```python
from build123d import *

# Parameters (mm, degrees)
BRIDA_BASE1_DEPTH         = 4
TALADRO_ROSCADO_M51_D     = 4.2
TALADRO_ROSCADO_M51_DEPTH = 14
TALADRO_ROSCADO_M51_TIP   = 1.2618073


# Sheet-metal steps are written as plain solids
with BuildPart() as part:
    # Croquis1 → Brida base1 (new body)
    with BuildSketch(Plane.XY):
        with BuildLine():
            Line((-19.990811444, 8), (-3.990811444, 8))
            ThreePointArc((-3.990811444, 8), (4.009188556, 0), (-3.990811444, -8))
            Line((-3.990811444, -8), (-19.990811444, -8))
            ThreePointArc((-19.990811444, -8), (-27.990811444, 0), (-19.990811444, 8))
        make_face()
    extrude(amount=-BRIDA_BASE1_DEPTH)

    # Taladro roscado M51
    with Locations(Plane.XY):
        with Locations((-19.990811444, 0), (-3.990811444, 0)):
            Hole(TALADRO_ROSCADO_M51_D / 2, depth=TALADRO_ROSCADO_M51_DEPTH)
            with Locations((0, 0, -(TALADRO_ROSCADO_M51_DEPTH + TALADRO_ROSCADO_M51_TIP / 2))):  # 118° drill point
                Cone(0, TALADRO_ROSCADO_M51_D / 2, TALADRO_ROSCADO_M51_TIP, mode=Mode.SUBTRACT)


solid = part.part
```
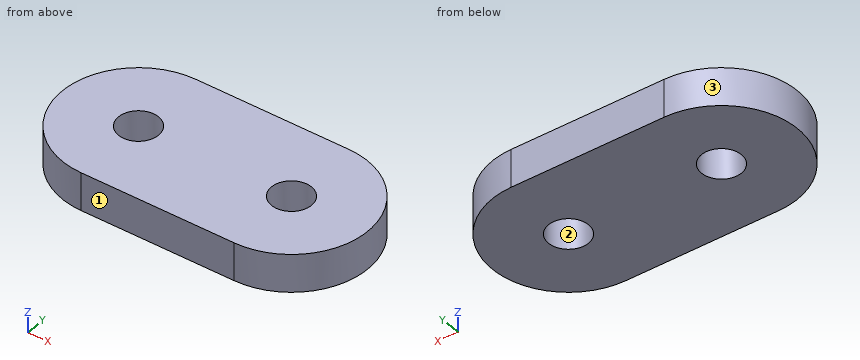
The model under review builds one solid part; all positions refer to its coordinate system, in mm. Face numbers are marked on the shaded views. Give positions to 0.01 mm unless a question says otherwise; leave off trailing zeros. Write each loop counter-clockwise with the first axis right and the second up, starting at its lowest first coordinate (ties: lowest second). Pieces come first, ordered by that corner, then holes. Notation, with made-up numbers: M 72,49.25 L 105,49.25 A25 cw 105,85.25 Z; hole C 55,-0.75 d3. An arc over 180 degrees is marked long. Write each question's results on one line, items separated by ' | '. Start each with the question number.
1. Insertion check: pin 1 Ø5.5 at (x, y) = (-3.99, 0) entering from -Z; pin 2 Ø1 at (y, z) = (5, -3) entering from +X; pin 3 Ø1.5 at (y, z) = (5, -2.5) entering from +X. Each pin has a flat end and moves straight along its axis. Give the tip position at first contact, or say it passes through.
2. We need section D-D (x = -25.5). Write out the cut boundary in (y, z), and give its area (3 significant figures).
3. We need section C-C (x = -5.5). Write out the cut boundary in (y, z).
4. We need section A-A (y = 0). Write out the cut boundary in (x, z), and give its area (3 significant figures).
5. Mouldability with a two-part tool opening along X and no side actions: class the marked faces 1, 2 and 3 as released by +X, released by -X, zero draft, split by the parting line, or undercut.
6. For probe 1 along X at (y, z) = (-0.75, -2.1); probe 2 along Y at (x, z) = (-19.5, -3.6); probe 3 along X at (y, z) = (7, -1.25), list the stretches that pass through material, from the lowest coordinate up. Write a range as [from, to].
7. We need section B-B (z = -2.7). Write out the cut boundary in (x, y), and give its area (3 significant figures).
Results found:
1) pin 1: stops at z = -4 | pin 2: stops at x = 2.62 | pin 3: stops at x = 2.79
2) outline: M -5.8,-4 L 5.8,-4 L 5.8,0 L -5.8,0 Z | area: 46.4 mm^2
3) outline: M -8,-4 L -1.46,-4 L -1.46,0 L -8,0 Z; M 1.46,-4 L 8,-4 L 8,0 L 1.46,0 Z
4) outline: M -27.99,-4 L -22.09,-4 L -22.09,0 L -27.99,0 Z; M -17.89,-4 L -6.09,-4 L -6.09,0 L -17.89,0 Z; M -1.89,-4 L 4.01,-4 L 4.01,0 L -1.89,0 Z | area: 94.4 mm^2
5) face 1: zero draft | face 2: undercut | face 3: released by -X
6) probe 1: x = [-27.96, -21.95], [-18.03, -5.95], [-2.03, 3.97] | probe 2: y = [-8, -2.04], [2.04, 8] | probe 3: x = [-23.86, -0.12]
7) outline: M -19.99,-8 L -3.99,-8 A8 ccw -3.99,8 L -19.99,8 A8 ccw Z; hole C -19.99,0 d4.2; hole C -3.99,0 d4.2 | area: 429 mm^2
